Input: dimensioned drawing with shaded views. Units: mm. Origin: part minimum x, y, z. A direction names the side the tool comes from. Round coordinates to 2 decimals unless told otherwise and drop trailing zeros. Order: outer loops, then holes, each group sorted by start corner. A loop starts at its lowest first (then second) coordinate and runs counter-clockwise, first axis right, second up. Notation, with made-up numbers: (-36.5, -16) - (-15.5, -16) arc R15 cw to (-15.5, 9) - close; hole circle Ø5 at (-10, 62.5). An arc over 180 degrees is marked (long way). Put each result on its own line as item: value. Start each with the question number.
(1) Section C-C (z = 20). Output: boundary loops of the cut face in (x, y) (3 decimals).
(2) Pin query (flat end, axial travel): P1, Ø3, axis at y = 5.5, z = 20, coming from the +X side; P2, Ø1, axis at y = 3.5, z = 7, coming from the -X side; P3, Ø5.5, axis at x = 26, z = 12.5, coming from the +Y side (3 decimals); P4, Ø4, axis at x = 31.75, z = 6.35, coming from the +Y side. Return the tip coordinate at first contact, or that it passes through.
(3) Section A-A (x = 31.75). Output: boundary loops of the cut face in (y, z) (3 decimals).
(4) Section D-D (x = 8.89). Output: boundary loops of the cut face in (y, z) (3 decimals).
(5) Section B-B (y = 7). Output: boundary loops of the cut face in (x, z) (3 decimals).
(6) Access query for the marked faces 4 and 5. Directions: +Z, -Z, +X, -X, +Y, -Y. A direction counts if a zero-diameter tool reaches every point of the face in a straight line with its end or side. Return the directions, or none.
(7) Material intervals for L1, parallel to Z at x = 31.75, y = 1.6 (3 decimals); L2, parallel to X at y = 1.8, z = 31.75 (3 decimals); L3, parallel to X at y = 8, z = 26.5 (3 decimals), sorted ascending. Write a range as [from, to].
(8) Pull-direction query (Z, two-part tool) for the marked faces 1, 2 and 3; classes: released by +Z, released by -Z, zero draft, split by the parting line, or undercut.
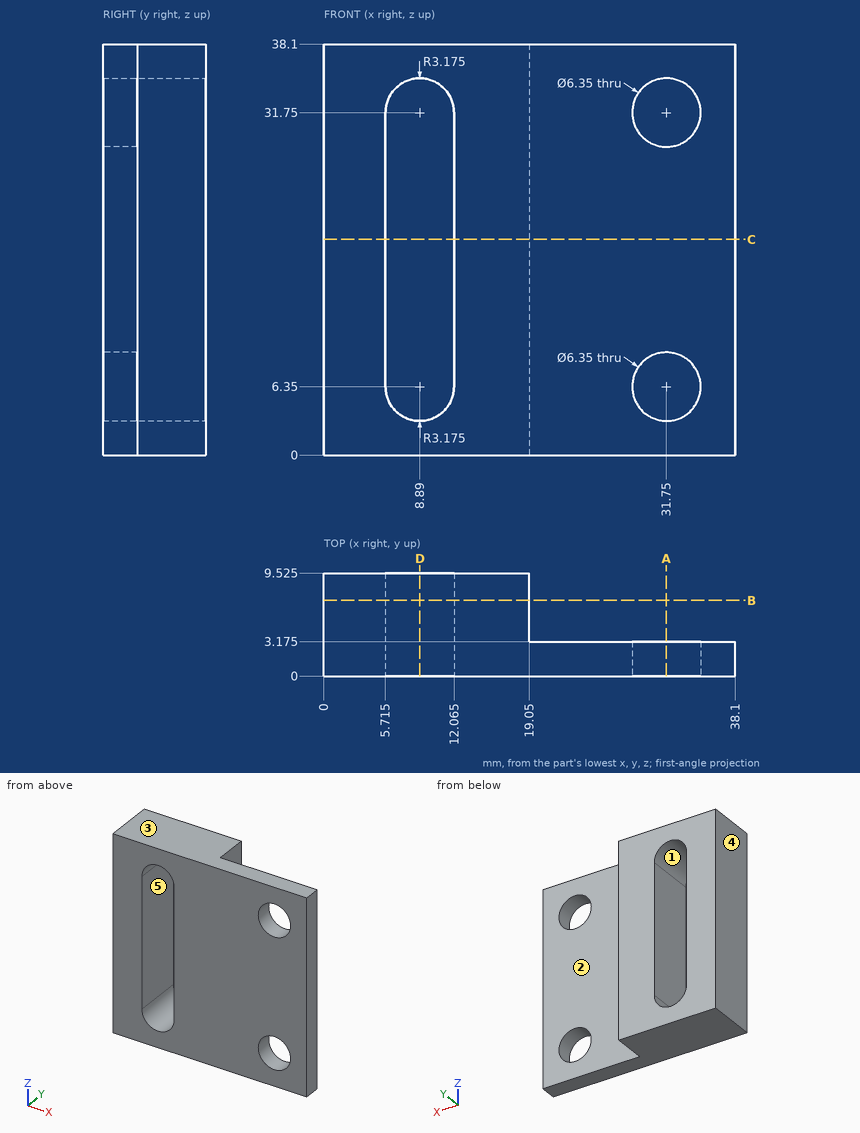
Checks:
1. outline: (0, 0) - (5.715, 0) - (5.715, 9.525) - (0, 9.525) - close; (12.065, 0) - (38.1, 0) - (38.1, 3.175) - (19.05, 3.175) - (19.05, 9.525) - (12.065, 9.525) - close
2. P1: stops at x = 19.05
2. P2: stops at x = 0
2. P3: stops at y = 3.175
2. P4: passes through
3. outline: (0, 0) - (3.175, 0) - (3.175, 3.175) - (0, 3.175) - close; (0, 9.525) - (3.175, 9.525) - (3.175, 28.575) - (0, 28.575) - close; (0, 34.925) - (3.175, 34.925) - (3.175, 38.1) - (0, 38.1) - close
4. outline: (0, 0) - (9.525, 0) - (9.525, 3.175) - (0, 3.175) - close; (0, 34.925) - (9.525, 34.925) - (9.525, 38.1) - (0, 38.1) - close
5. outline: (0, 0) - (19.05, 0) - (19.05, 38.1) - (0, 38.1) - close; hole (5.715, 6.35) arc R3.175 ccw to (12.065, 6.35) - (12.065, 31.75) arc R3.175 ccw to (5.715, 31.75) - close
6. face 4: +Z, -Z, -X, +Y, -Y
6. face 5: +Y, -Y
7. L1: z = [0, 3.175], [9.525, 28.575], [34.925, 38.1]
7. L2: x = [0, 5.715], [12.065, 28.575], [34.925, 38.1]
7. L3: x = [0, 5.715], [12.065, 19.05]
8. face 1: undercut
8. face 2: zero draft
8. face 3: released by +Z
